Geometry check sheet. Reference: drawing and pictorial views, mm from the part's lowest x, y, z. A direction names the side the tool comes from. Round coordinates to 2 decimals unless told otherwise and drop trailing zeros. Order: outer loops, then holes, each group sorted by start corner. A loop starts at its lowest first (then second) coordinate and runs counter-clockwise, first axis right, second up. Notation, with made-up numbers: (38.5, 72.5) -> (96.5, 72.5) arc R30 cw to (96.5, 98.5) -> close; hole circle Ø3 at (-11, 35.5). An arc over 180 degrees is marked (long way). Put each result on its own line as item: value.
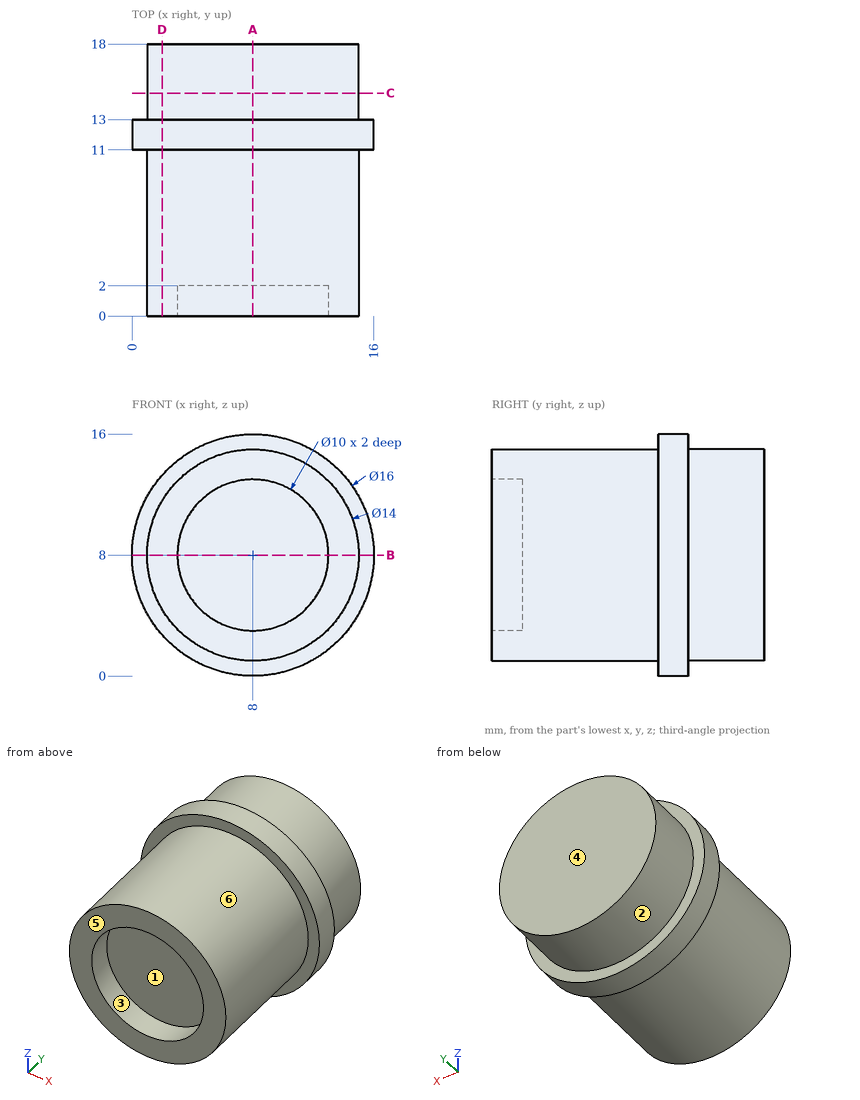
Item 1: Sectioned sample at C-C, the plane y = 14.75. Record the boundary of the cut face in (x, z), then the cut area to 3 significant figures.
Geometry check:
outline: circle Ø14 at (8, 8)
area: 154 mm2
Item 2: Sectioned sample at A-A, the plane x = 8. Record the boundary of the cut face in (y, z), then the cut area to 3 significant figures.
Geometry check:
outline: (0, 1) -> (11, 1) -> (11, 0) -> (13, 0) -> (13, 1) -> (18, 1) -> (18, 15) -> (13, 15) -> (13, 16) -> (11, 16) -> (11, 15) -> (0, 15) -> (0, 13) -> (2, 13) -> (2, 3) -> (0, 3) -> close
area: 236 mm2
Item 3: Material ranges on line 1 along Z through (x, y) = (8, 0.85); line 2 along Y through (x, z) = (6.5, 7.25); line 3 along Z through (x, y) = (8.75, 8.25), recorded low to high.
Geometry check:
line 1: 1 to 3, 13 to 15
line 2: 2 to 18
line 3: 1.04 to 14.96
Item 4: Sectioned sample at B-B, the plane z = 8. Record the boundary of the cut face in (x, y), then the cut area to 3 significant figures.
Geometry check:
outline: (0, 11) -> (1, 11) -> (1, 0) -> (3, 0) -> (3, 2) -> (13, 2) -> (13, 0) -> (15, 0) -> (15, 11) -> (16, 11) -> (16, 13) -> (15, 13) -> (15, 18) -> (1, 18) -> (1, 13) -> (0, 13) -> close
area: 236 mm2
Item 5: Sectioned sample at D-D, the plane x = 2. Record the boundary of the cut face in (y, z).
Geometry check:
outline: (0, 4.39) -> (11, 4.39) -> (11, 2.71) -> (13, 2.71) -> (13, 4.39) -> (18, 4.39) -> (18, 11.61) -> (13, 11.61) -> (13, 13.29) -> (11, 13.29) -> (11, 11.61) -> (0, 11.61) -> close
Item 6: Release check for a two-part mould opening along Z. For the marked faces 1, 2, 3 and 4 record: pulls with the +Z half, pulls with the -Z half, needs draft (parallel to the pull), parting line crosses it, or undercut.
Geometry check:
face 1: undercut
face 2: parting line crosses it
face 3: undercut
face 4: needs draft
Item 7: Depth check by flat-ended pin: pin 1 Ø4 at (x, y) = (5, 12.5) entering from -Z; pin 2 Ø1 at (x, y) = (2, 15.5) entering from -Z; pin 3 Ø2 at (x, z) = (13, 3) entering from -Y; pin 4 Ø5 at (x, z) = (7.5, 6.5) entering from -Y. Enter the tip coordinate at first touch or a pass-through.
Geometry check:
pin 1: z = 0.06
pin 2: z = 3.67
pin 3: y = 0
pin 4: y = 2
Item 8: Tool access check on the marked faces 5 and 6. Record the directions out of +Z, -Z, +X, -X, +Y, -Y that give a thin tool (end or side, any length) a straight path to the whole face; none if there is none.
Geometry check:
face 5: +Z, -Z, +X, -X, -Y
face 6: -Y
